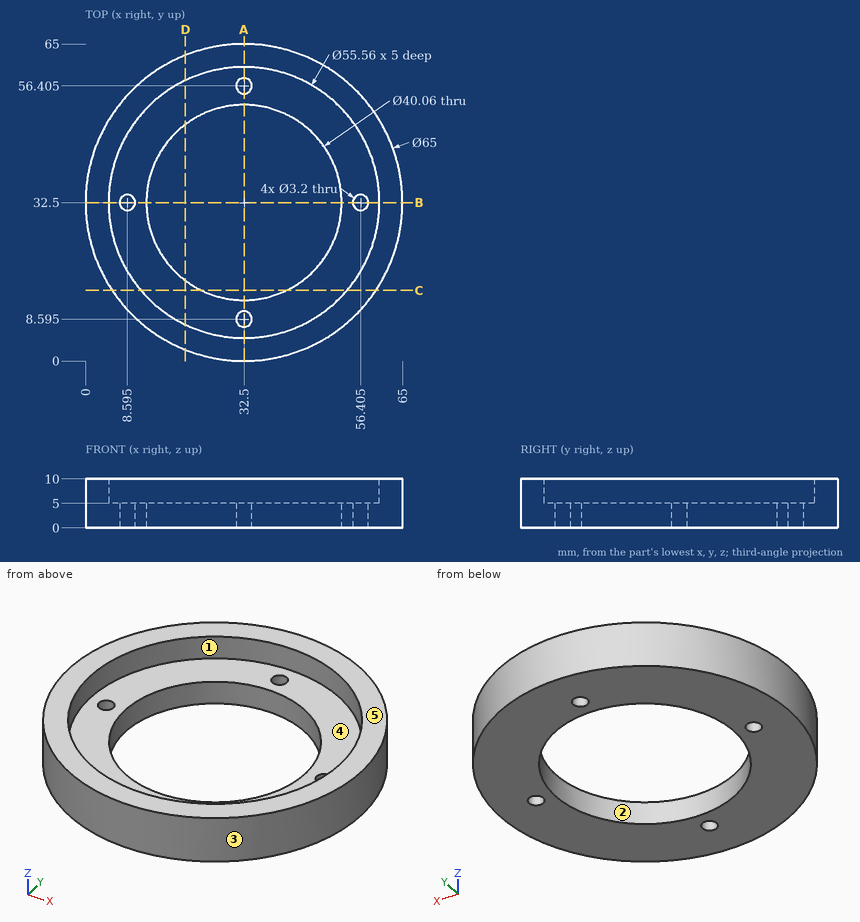
Study the drawing (mm; zero at the part's minimum x, y, z) and answer. A direction names the side the tool comes from. Coordinates: 2 decimals unless noted, no trailing zeros. Write each loop counter-clockwise with the first axis right and the second up, starting at its lowest first coordinate (ties: lowest second). Pieces come first, ordered by that corner, then holes.
Q1. Each of these flat-tipped pins is pushed along its axis until it touches: pin 1 Ø1 at (x, z) = (55, 7.5) entering from +Y; pin 2 Ø6 at (x, z) = (39.5, 3) entering from +Y; pin 3 Ø5 at (y, z) = (25.5, 1.5) entering from +X. Where does it stop, or does it pass through?
Q2. Which of the six approach directions +Z, -Z, +X, -X, +Y, -Y give full straight-line access (tool end or side, diameter ignored) to the marked faces 1 and 2?
Q3. A cutting plane is placed at A-A, the plane x = 32.5. Give the vertices of the cut face in (y, z) (3 decimals).
Q4. Find the intervals of material crossed by line 1 (X direction, y = 31.5, z = 2.5); line 2 (X direction, y = 27.5, z = 3); line 3 (Y direction, x = 49.5, z = 8), in increasing order.
Q5. A cutting plane is placed at C-C, the plane y = 14.5. Give the vertices of the cut face in (x, z).
Q6. A cutting plane is placed at D-D, the plane x = 20.5. Give the vertices of the cut face in (y, z), then the cut area to 3 significant figures.
Q7. Determine the mould class of the marked faces 3, 4 and 5 for opening direction Y: released by +Y, released by -Y, zero draft, split by the parting line, or undercut.
Findings below:
1. pin 1: stops at y = 56.42
1. pin 2: stops at y = 64.75
1. pin 3: stops at x = 64.69
2. face 1: +Z
2. face 2: +Z, -Z
3. outline: (0, 0) - (6.995, 0) - (6.995, 5) - (4.72, 5) - (4.72, 10) - (0, 10) - close; (10.195, 0) - (12.47, 0) - (12.47, 5) - (10.195, 5) - close; (52.53, 0) - (54.805, 0) - (54.805, 5) - (52.53, 5) - close; (58.005, 0) - (65, 0) - (65, 10) - (60.28, 10) - (60.28, 5) - (58.005, 5) - close
4. line 1: x = 0.02 to 7.35, 9.84 to 12.49, 52.51 to 55.16, 57.65 to 64.98
4. line 2: x = 0.39 to 13.1, 51.9 to 64.61
4. line 3: y = 4.8 to 10.53, 54.47 to 60.2
5. outline: (5.44, 0) - (23.71, 0) - (23.71, 5) - (11.34, 5) - (11.34, 10) - (5.44, 10) - close; (41.29, 0) - (59.56, 0) - (59.56, 10) - (53.66, 10) - (53.66, 5) - (41.29, 5) - close
6. outline: (2.3, 0) - (16.46, 0) - (16.46, 5) - (7.45, 5) - (7.45, 10) - (2.3, 10) - close; (48.54, 0) - (62.7, 0) - (62.7, 10) - (57.55, 10) - (57.55, 5) - (48.54, 5) - close
6. area: 193 mm2
7. face 3: split by the parting line
7. face 4: undercut
7. face 5: zero draft
